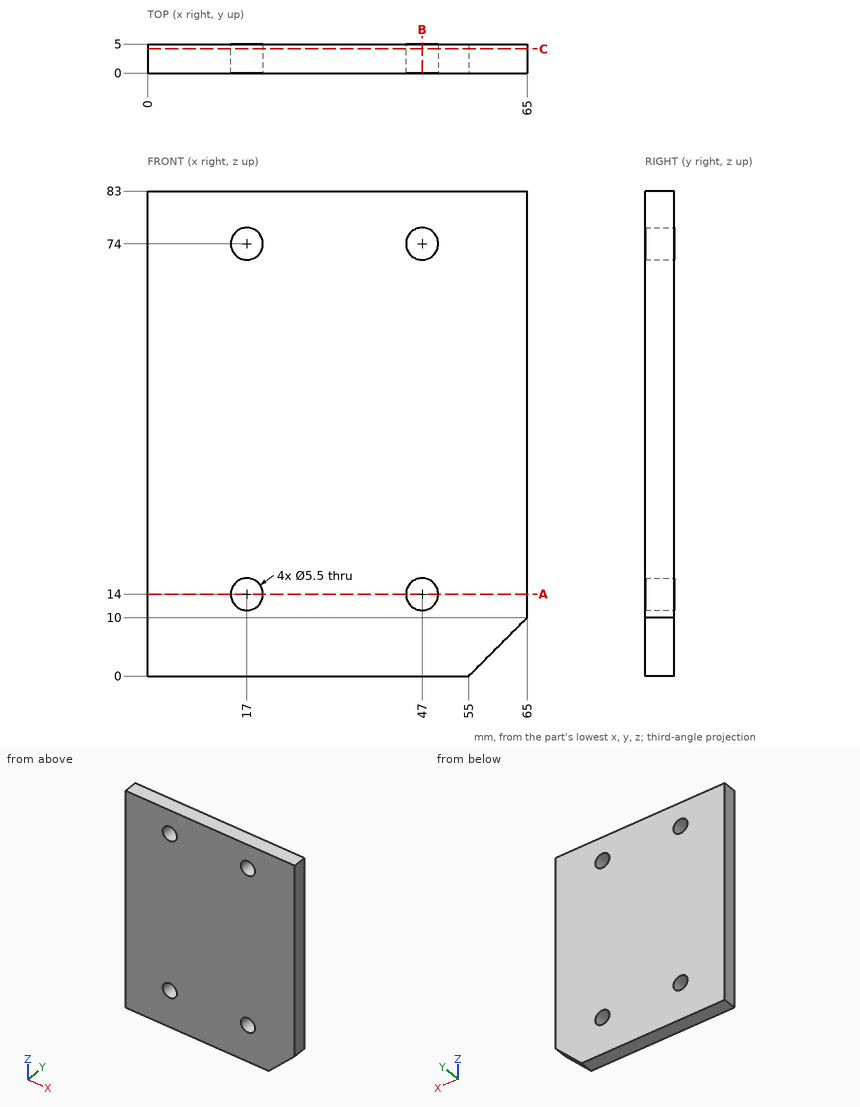
The drawing under review shows one solid part. Ordinate dimensions are in mm from its lowest x, y, z. Round coordinates to 2 decimals unless told otherwise and drop trailing zeros. Order: outer loops, then holes, each group sorted by start corner. A loop starts at its lowest first (then second) coordinate and runs counter-clockwise, first axis right, second up. Notation, with made-up numbers: (57.25, -36) - (84.25, -36) arc R29 ccw to (84.25, 1) - close; hole circle Ø6 at (32, 30.25). An arc over 180 degrees is marked (long way). Return JSON: item names as keys, results as strings.
Q1. Consider section B-B on x = 47. Write out the cut boundary in (y, z).
Computed values:
{"outline": "(0, 0) - (5, 0) - (5, 11.25) - (0, 11.25) - close; (0, 16.75) - (5, 16.75) - (5, 71.25) - (0, 71.25) - close; (0, 76.75) - (5, 76.75) - (5, 83) - (0, 83) - close"}
Q2. Consider section C-C on y = 4.15. Write out the cut boundary in (x, z).
Computed values:
{"outline": "(0, 0) - (55, 0) - (65, 10) - (65, 83) - (0, 83) - close; hole circle Ø5.5 at (17, 14); hole circle Ø5.5 at (17, 74); hole circle Ø5.5 at (47, 14); hole circle Ø5.5 at (47, 74)"}
Q3. Consider section A-A on z = 14. Write out the cut boundary in (x, y).
Computed values:
{"outline": "(0, 0) - (14.25, 0) - (14.25, 5) - (0, 5) - close; (19.75, 0) - (44.25, 0) - (44.25, 5) - (19.75, 5) - close; (49.75, 0) - (65, 0) - (65, 5) - (49.75, 5) - close"}
Q4. For pin 1 Ø4.5 at (x, z) = (47, 74) entering from +Y, flat-tipped, find the tip position at first contact; note if it passes through.
Computed values:
{"pin 1": "passes through"}
Q5. Wall thickness on L1, parallel to Z at x = 17, y = 3.45; L2, parallel to Z at x = 48.5, y = 3.1; L3, parallel to X at y = 0.7, z = 11.5: over which ranges is each line inside the solid? List them lowest first. Write a range as [from, to].
Computed values:
{"L1": "z = [0, 11.25], [16.75, 71.25], [76.75, 83]", "L2": "z = [0, 11.7], [16.3, 71.7], [76.3, 83]", "L3": "x = [0, 15.85], [18.15, 45.85], [48.15, 65]"}
